Verification items for the finished model (mm, model axes). A direction names the side the tool comes from. Coordinates: 2 decimals unless noted, no trailing zeros. Write each loop counter-clockwise with the first axis right and the second up, starting at its lowest first coordinate (ties: lowest second). Pieces come first, ordered by that corner, then holes. Notation, with made-up numbers: (67, 16.25) -> (88, 16.25) arc R20 ccw to (88, 36.25) -> close; hole circle Ø8 at (68.5, -25.75). An arc over 180 degrees is marked (long way). Answer in a Markdown table with one row per item.
```python
from build123d import *

# Parameters (mm, degrees)
F2_R     = 1.1
F3_DEPTH = 8
F5_DEPTH = 1
F6_R     = 0.5


with BuildPart() as f1:
    # F0 (on Right) → F1 (revolve)
    with BuildSketch(Plane.YZ):
        with BuildLine():
            Line((-7, 0), (0, 0))
            Line((0, 0), (0, 10))
            Line((0, 10), (-5, 10))
            ThreePointArc((-5, 10), (-5.060069, 5.195667), (-7, 0.8))
            Line((-7, 0.8), (-7, 0))
        make_face()
    revolve(axis=Axis((0, 0, 7.262046), (0, 0, -1)))

    # F2 (on face) → F3 (cut)
    with BuildSketch(Plane(origin=(0, 0, 0), x_dir=(1, 0, 0), z_dir=(0, 0, -1))):
        Circle(F2_R)
    extrude(amount=-F3_DEPTH, mode=Mode.SUBTRACT)

    # F4 (on face) → F5 (cut)
    with BuildSketch(Plane.XY.offset(10)):
        with BuildLine():
            Line((-0.5, 0.5), (-0.5, 3.968627))
            ThreePointArc((-0.5, 3.968627), (-2.828427, 2.828427), (-3.968627, 0.5))
            Line((-3.968627, 0.5), (-0.5, 0.5))
        make_face()
        with BuildLine():
            ThreePointArc((3.968627, 0.5), (2.828427, 2.828427), (0.5, 3.968627))
            Line((0.5, 3.968627), (0.5, 0.5))
            Line((0.5, 0.5), (3.968627, 0.5))
        make_face()
        with BuildLine():
            Line((-0.5, -0.5), (-3.968627, -0.5))
            ThreePointArc((-3.968627, -0.5), (-2.828427, -2.828427), (-0.5, -3.968627))
            Line((-0.5, -3.968627), (-0.5, -0.5))
        make_face()
        with BuildLine():
            Line((0.5, -0.5), (0.5, -3.968627))
            ThreePointArc((0.5, -3.968627), (2.828427, -2.828427), (3.968627, -0.5))
            Line((3.968627, -0.5), (0.5, -0.5))
        make_face()
    extrude(amount=-F5_DEPTH, mode=Mode.SUBTRACT)

    # F6
    f6_edges = [f1.edges().sort_by_distance(p)[0] for p in [
        (-2.234313, 0.5, 9),
        (-0.5, 2.234313, 9),
        (-2.828427, 2.828427, 9),
        (2.828427, 2.828427, 9),
        (0.5, 2.234313, 9),
        (2.234313, 0.5, 9),
        (2.234313, -0.5, 9),
        (0.5, -2.234313, 9),
        (2.828427, -2.828427, 9),
        (-0.5, -2.234313, 9),
        (-2.234313, -0.5, 9),
        (-2.828427, -2.828427, 9),
    ]]
    fillet(f6_edges, radius=F6_R)


solid = f1.part
```
1. Release check for a two-part mould opening along Y. For faces 1 (the face through (0, 0, 10)), 2 (the face through (2, -2, 9)), 3 (the face through (1.05, -0.33, 3.94)), 4 (the face through (2.681, -6.466, 0.394)) record: released by +Y, released by -Y, zero draft, split by the parting line, or undercut.
Findings below:
| item | result |
|---|---|
| face 1 | zero draft |
| face 2 | undercut |
| face 3 | undercut |
| face 4 | split by the parting line |
2. Sectioned sample at D-D, the plane z = 1. Record the cut outline in (x, y), and give its area (3 significant figures).
Findings below:
| item | result |
|---|---|
| outline | circle Ø13.72 at (0, 0); hole circle Ø2.2 at (0, 0) |
| area | 144 mm² |
3. Material ranges on probe 1 along Z at (x, y) = (2.5, 2); probe 2 along Y at (x, z) = (0, 2); probe 3 along Y at (x, z) = (0, 6.25), recorded low to high. Write a range as from..to.
Findings below:
| item | result |
|---|---|
| probe 1 | z = 0..9 |
| probe 2 | y = -6.25..-1.1, 1.1..6.25 |
| probe 3 | y = -4.88..-1.1, 1.1..4.88 |
4. Sectioned sample at A-A, the plane y = 0. Record the cut outline in (x, z).
Findings below:
| item | result |
|---|---|
| outline | (-7, 0) -> (-1.1, 0) -> (-1.1, 8) -> (1.1, 8) -> (1.1, 0) -> (7, 0) -> (7, 0.8) arc R12 cw to (5, 10) -> (-5, 10) arc R12 cw to (-7, 0.8) -> close |
5. Sectioned sample at C-C, the plane z = 3.75. Record the cut outline in (x, y).
Findings below:
| item | result |
|---|---|
| outline | circle Ø10.94 at (0, 0); hole circle Ø2.2 at (0, 0) |
6. Access from +Z, -Z, +X, -X, +Y, -Y to the whole of each face (thin tool, end or side, straight path). Record for faces 5 (the face through (-2, -2, 9)), 6 (the face through (1.5, 0.1, 0)), 7 (the face through (0, 0, 8)).
Findings below:
| item | result |
|---|---|
| face 5 | +Z |
| face 6 | -Z, +X, -X, +Y, -Y |
| face 7 | -Z |
7. Go/stop test with flat-tipped pins: pin 1 (3 mm diameter, centred on x = 0, z = 5.5, fed in from +Y); pin 2 (1 mm diameter, centred on y = -1.5, z = 2, fed in from -X); pin 3 (4 mm diameter, centred on x = 5.5, z = 3.5, fed in from -Y). Record where each tip stops, or that it passes through.
Findings below:
| item | result |
|---|---|
| pin 1 | stops at y = 5.39 |
| pin 2 | stops at x = -6.38 |
| pin 3 | stops at y = -4.68 |
